Can you work these out from the model? Positions are in its coordinate system, mm. A direction names the side the tool comes from. Give positions to 0.01 mm unless a question says otherwise; leave off trailing zeros. Loops run counter-clockwise (first coordinate to the right, second up) from the corner with the lowest first, then second, coordinate; pieces in that order, holes last. Notation, with made-up numbers: (68, -4) - (124, -4) arc R23 ccw to (124, 14) - close; hole circle Ø3 at (-24, 41). An arc over 180 degrees is marked (long way). Write item = value, one per line.
from build123d import *

# Parameters (mm, degrees)
F1_DEPTH = 4
F2_W     = 4
F2_H     = 12
F3_DEPTH = 22
F5_DEPTH = 25
F7_DEPTH = 1.5
F8_R     = 5


# Not quite as in the source:
# - a feature names something its author has since deleted; it is built from what else it names


with BuildPart() as f1:
    # F0 (on Top) → F1 (new body)
    with BuildSketch(Plane.XY):
        with BuildLine():
            ThreePointArc((0, -3), (-0.8786796564, -0.8786796564), (-3, 0))
            Line((-3, 0), (-23, 0))
            Line((-23, 0), (-23, -12))
            Line((-23, -12), (-3, -12))
            ThreePointArc((-3, -12), (-0.8786796564, -11.1213203436), (0, -9))
            Line((0, -9), (0, -3))
        make_face()
        with BuildLine():
            ThreePointArc((-3, -3.95), (-0.95, -6), (-3, -8.05))
            Line((-3, -8.05), (-14, -8.05))
            ThreePointArc((-14, -8.05), (-16.05, -6), (-14, -3.95))
            Line((-14, -3.95), (-3, -3.95))
        make_face(mode=Mode.SUBTRACT)
    extrude(amount=F1_DEPTH)

    # F2 (on face) → F3 (join)
    with BuildSketch(Plane.XY.offset(4)):
        with Locations((-21, -6)):
            Rectangle(F2_W, F2_H)
    extrude(amount=F3_DEPTH)

    # F4 (on face) → F5 (cut)
    with BuildSketch(Plane(origin=(-23, 0, 0), x_dir=(0, -1, 0), z_dir=(-1, 0, 0))):
        with BuildLine():
            Line((4, 21), (4, 9))
            ThreePointArc((4, 9), (4.5857864376, 7.5857864376), (6, 7))
            ThreePointArc((6, 7), (7.4142135624, 7.5857864376), (8, 9))
            Line((8, 9), (8, 21))
            ThreePointArc((8, 21), (7.4142135624, 22.4142135624), (6, 23))
            ThreePointArc((6, 23), (4.5857864376, 22.4142135624), (4, 21))
        make_face()
    extrude(amount=-F5_DEPTH, mode=Mode.SUBTRACT)

    # F6 (on face) → F7 (cut)
    with BuildSketch(Plane.YZ.offset(-19)):
        Polygon((-6, 4.8430780618), (-2.4, 6.9215390309), (-2.4, 23.0784609691), (-6, 25.1569219382), (-9.6, 23.0784609691), (-9.6, 6.9215390309), align=None)
        with BuildLine():
            ThreePointArc((-8, 21), (-6, 23), (-4, 21))
            Line((-4, 21), (-4, 9))
            ThreePointArc((-4, 9), (-6, 7), (-8, 9))
            Line((-8, 9), (-8, 21))
        make_face(mode=Mode.SUBTRACT)
    extrude(amount=-F7_DEPTH, mode=Mode.SUBTRACT)

    # F8
    f8_edges = [f1.edges().sort_by_distance(p)[0] for p in [
        (-21, -12, 26),
        (-21, 0, 26),
    ]]
    fillet(f8_edges, radius=F8_R)


solid = f1.part
Q1. We'd pull the mould along Z, two halves only. Please class faces 4 (the cylindrical face through (-21, -2, 25)), 5 (the flat face through (-22, -4, 15)), 6 (the flat face through (-9, -3.95, 2)): released by +Z, released by -Z, zero draft, split by the parting line, or undercut.
Output:
face_4 = released by +Z
face_5 = undercut
face_6 = zero draft
Q2. Imagine slicing it at D-D, the plane y = -10. Write out the boundary of the cut face in (x, z).
Output:
outline = (-23, 0) - (-0.17, 0) - (-0.17, 4) - (-19, 4) - (-19, 25) - (-23, 25) - close
Q3. I need wall thicknesses on L1, parallel to Y at x = -12.25, z = 1.5; L2, parallel to Z at x = -5.75, y = -2; L3, parallel to X at y = -3.75, z = 5.25. Which ranges of each line are inside material? Lowest first, please.
Output:
L1 = -12 to -8.05, -3.95 to 0
L2 = 0 to 4
L3 = -23 to -19
Q4. Imagine slicing it at B-B, the plane z = 16.25. Write out the boundary of the cut face in (x, y).
Output:
outline = (-23, -12) - (-19, -12) - (-19, -9.6) - (-20.5, -9.6) - (-20.5, -8) - (-23, -8) - close; (-23, -4) - (-20.5, -4) - (-20.5, -2.4) - (-19, -2.4) - (-19, 0) - (-23, 0) - close
Q5. For pin 1 (5 mm diameter, centred on y = -4.5, z = 14, fed in from +X); pin 2 (3 mm diameter, centred on x = -16, y = -8, fed in from +Z), each with a flat end and sliding along its axis, tell me the tip position at first contact or that it passes through.
Output:
pin_1 = -19
pin_2 = 4
Q6. Which directions (+Z, -Z, +X, -X, +Y, -Y) give clear straight access to the entire face, cutting with the end or side of a thin tool? Please do faces 1 (the flat face through (-8, -8.05, 2)), 2 (the flat face through (-20, -8, 6)), 3 (the flat face through (-22, -8, 15)).
Output:
face_1 = +Z, -Z
face_2 = +X
face_3 = +X, -X
Q7. Imagine slicing it at A-A, the plane x = -12. Write out the boundary of the cut face in (y, z), then the cut area to 3 significant figures.
Output:
outline = (-12, 0) - (-8.05, 0) - (-8.05, 4) - (-12, 4) - close; (-3.95, 0) - (0, 0) - (0, 4) - (-3.95, 4) - close
area = 31.6 mm2
Q8. Imagine slicing it at C-C, the plane z = 2. Write out the boundary of the cut face in (x, y).
Output:
outline = (-23, -12) - (-3, -12) arc R3 ccw to (0, -9) - (0, -3) arc R3 ccw to (-3, 0) - (-23, 0) - close; hole (-14, -8.05) - (-3, -8.05) arc R2.05 ccw to (-3, -3.95) - (-14, -3.95) arc R2.05 ccw to start
